```python
from build123d import *

# Parameters (mm, degrees)
F0_R     = 50.8
F1_DEPTH = 82.55
F2_T     = -2.54
F5_DEPTH = 152.4


# Not quite as in the source:
# - a fillet or chamfer that OpenCascade refuses, or shapes differently, is made with other operations: its cross-section is extruded or revolved along the edge and cut away or added


with BuildPart() as f1:
    # F0 (on Right) → F1 (new body, symmetric)
    with BuildSketch(Plane.YZ):
        Circle(F0_R)
    extrude(amount=F1_DEPTH, both=True)

    # F2
    f2_openings = [f1.faces().sort_by_distance(p)[0] for p in [
        (82.55, 0, 0),
    ]]
    offset(amount=F2_T, openings=f2_openings)

    # F3: fillet of radius 5.08 on 3 edges, made by hand

    # F3_s1 → F3_t2 (revolve, cut)
    with BuildSketch(Plane.XY):
        with BuildLine():
            ThreePointArc((-77.47, 50.8), (-81.0621024484, 49.3121024484), (-82.55, 45.72))
            Line((-82.55, 45.72), (-82.55, 50.8))
            Line((-82.55, 50.8), (-77.47, 50.8))
        make_face()
    revolve(axis=Axis((-82.55, 0, 0), (1, 0, 0)), mode=Mode.SUBTRACT)

    # F3_s3 → F3_t4 (revolve, cut)
    with BuildSketch(Plane.XY):
        with BuildLine():
            ThreePointArc((78.1505909488, 50.8), (80.6905909488, 50.1194090512), (82.55, 48.26))
            Line((82.55, 48.26), (82.55, 50.8))
            Line((82.55, 50.8), (78.1505909488, 50.8))
        make_face()
    revolve(axis=Axis((82.55, 0, 0), (1, 0, 0)), mode=Mode.SUBTRACT)

    # F4 (on Top) → F5 (cut)
    with BuildSketch(Plane.XY):
        Polygon((-53.9159391403, 0), (-53.9159391403, 41.275), (-66.6159391403, 41.275), (-66.6159391403, 0), (-66.6159391403, -41.275), (-53.9159391403, -41.275), align=None)
    extrude(amount=F5_DEPTH, mode=Mode.SUBTRACT)


solid = f1.part
```
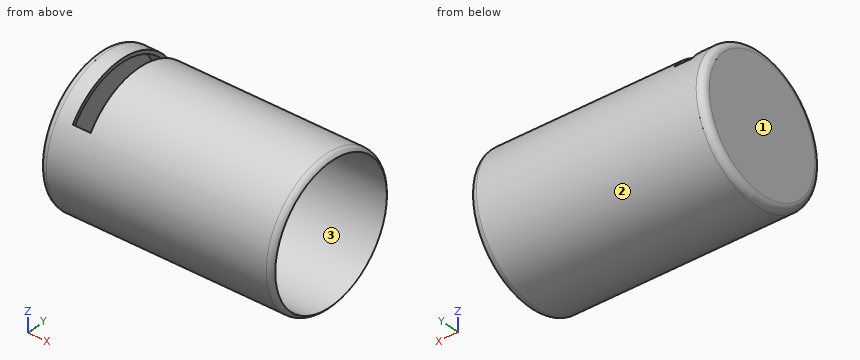
Work out the finished part from the listing and answer in its coordinate system (mm). Face numbers are marked on the shaded views. Coordinates: 2 decimals unless noted, no trailing zeros. Write each loop counter-clockwise with the first axis right and the second up, starting at its lowest first coordinate (ties: lowest second). Pieces come first, ordered by that corner, then holes.
Q1. A cutting plane is placed at C-C, the plane x = 53. Give the vertices of the cut face in (y, z), then the cut area to 3 significant figures.
Q2. A cutting plane is placed at A-A, the plane y = 0. Give the vertices of the cut face in (x, z).
Q3. Find the intervals of material crossed by line 1 (Y direction, x = -59, z = -1); line 2 (Z direction, x = -4, y = 0); line 3 (X direction, y = -9, z = -15), in increasing order.
Q4. Each of these flat-tipped pins is pushed along its axis until it touches: pin 1 Ø6 at (y, z) = (6, 2) entering from +X; pin 2 Ø2 at (x, y) = (-29, 37.5) entering from -Z; pin 3 Ø2 at (x, y) = (41, -39) entering from +Z. Where does it stop, or does it pass through?
Q5. Determine the mould class of the marked faces 1, 2 and 3 for opening direction Y: released by +Y, released by -Y, zero draft, split by the parting line, or undercut.
Q6. A cutting plane is placed at B-B, the plane z = 0. Give the vertices of the cut face in (x, y).
Findings below:
1. outline: circle Ø101.6 at (0, 0); hole circle Ø96.52 at (0, 0)
1. area: 790 mm2
2. outline: (-82.55, -45.72) arc R5.08 ccw to (-77.47, -50.8) - (78.15, -50.8) arc R5.08 ccw to (82.55, -48.26) - (-80.01, -48.26) - (-80.01, 48.26) - (-66.62, 48.26) - (-66.62, 50.8) - (-77.47, 50.8) arc R5.08 ccw to (-82.55, 45.72) - close; (-53.92, 48.26) - (82.55, 48.26) arc R5.08 ccw to (78.15, 50.8) - (-53.92, 50.8) - close
3. line 1: y = -50.79 to -48.25, 48.25 to 50.79
3. line 2: z = -50.8 to -48.26, 48.26 to 50.8
3. line 3: x = -82.55 to -80.01
4. pin 1: stops at x = -80.01
4. pin 2: stops at z = -35.33
4. pin 3: stops at z = 33.71
5. face 1: zero draft
5. face 2: split by the parting line
5. face 3: undercut
6. outline: (-82.55, -45.72) arc R5.08 ccw to (-77.47, -50.8) - (78.15, -50.8) arc R5.08 ccw to (82.55, -48.26) - (-80.01, -48.26) - (-80.01, 48.26) - (82.55, 48.26) arc R5.08 ccw to (78.15, 50.8) - (-77.47, 50.8) arc R5.08 ccw to (-82.55, 45.72) - close
